Here's the drawing with two shaded views (mm, measured from the low corner). I have some questions. Coordinates: 2 decimals unless noted, no trailing zeros. Loops run counter-clockwise (first coordinate to the right, second up) from the corner with the lowest first, then second, coordinate; pieces in that order, holes last.
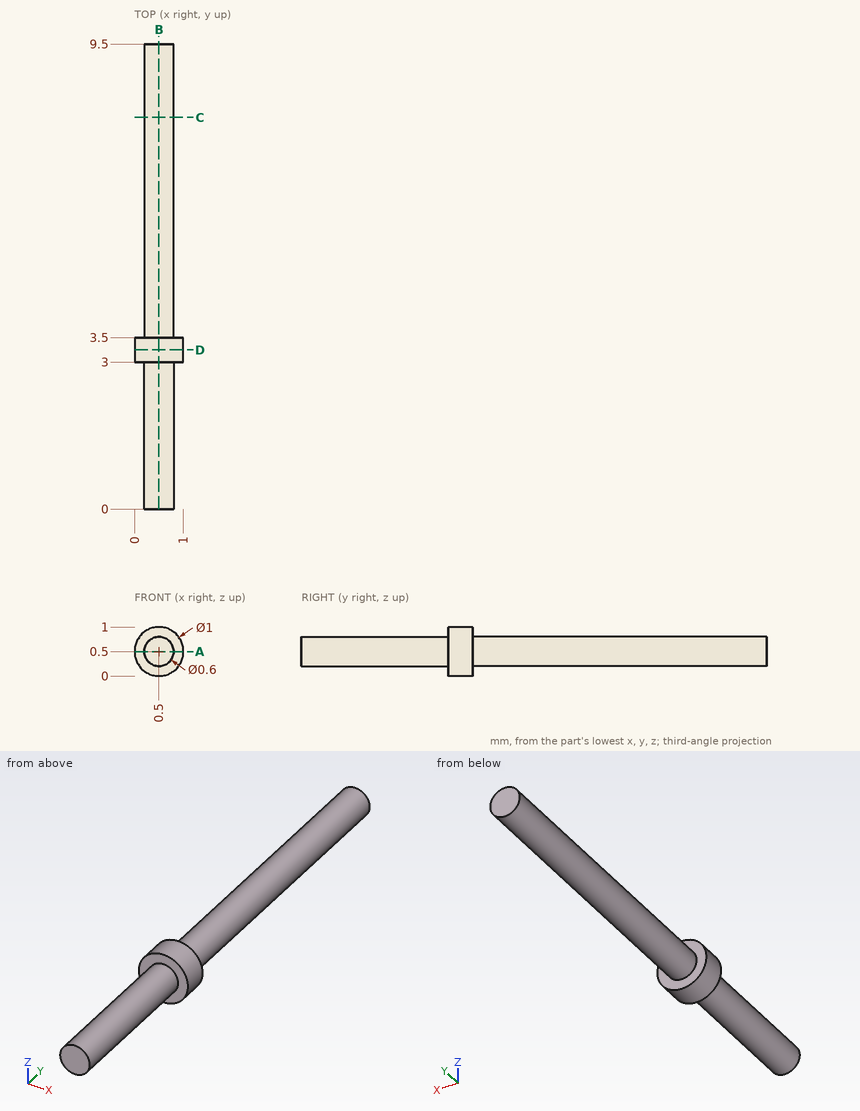
Q1. Suppose I cut it at C-C on y = 8. Write out the boundary of the cut face in (x, z), and give its area (3 significant figures).
Q2. Suppose I cut it at A-A on z = 0.5. Write out the boundary of the cut face in (x, y), and give its area (3 significant figures).
Q3. Suppose I cut it at D-D on y = 3.25. Write out the boundary of the cut face in (x, z), and give its area (3 significant figures).
Q4. Please list where these lines run through material, in increasing order: probe 1 along Y at (x, z) = (0.65, 0.8); probe 2 along Z at (x, y) = (0.5, 7); probe 3 along Z at (x, y) = (0.3, 8).
Q5. Suppose I cut it at B-B on x = 0.5. Write out the boundary of the cut face in (y, z), and give its area (3 significant figures).
Check values:
1. outline: circle Ø0.6 at (0.5, 0.5)
1. area: 0.283 mm2
2. outline: (0, 3) - (0.2, 3) - (0.2, 0) - (0.8, 0) - (0.8, 3) - (1, 3) - (1, 3.5) - (0.8, 3.5) - (0.8, 9.5) - (0.2, 9.5) - (0.2, 3.5) - (0, 3.5) - close
2. area: 5.90 mm2
3. outline: circle Ø1 at (0.5, 0.5)
3. area: 0.785 mm2
4. probe 1: y = 3 to 3.5
4. probe 2: z = 0.2 to 0.8
4. probe 3: z = 0.28 to 0.72
5. outline: (0, 0.2) - (3, 0.2) - (3, 0) - (3.5, 0) - (3.5, 0.2) - (9.5, 0.2) - (9.5, 0.8) - (3.5, 0.8) - (3.5, 1) - (3, 1) - (3, 0.8) - (0, 0.8) - close
5. area: 5.90 mm2
